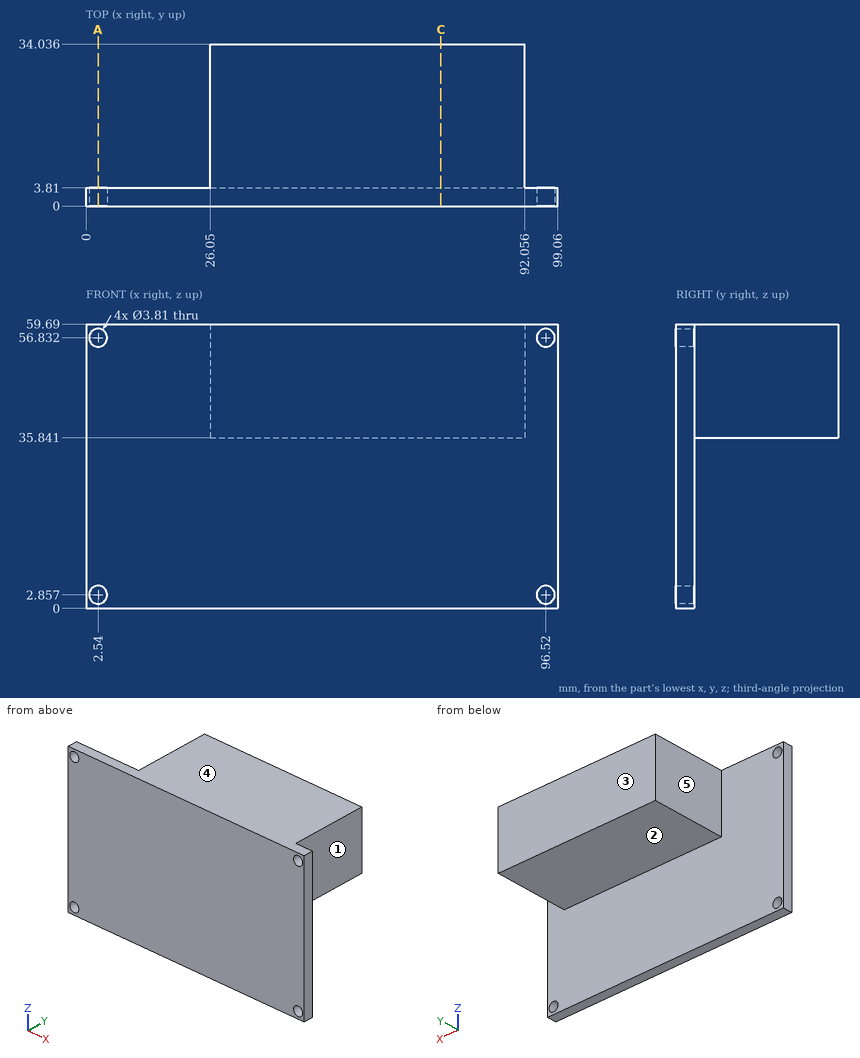
The figure shows three views and two pictorial views of one solid part (mm, origin at its lowest corner). Answer the questions. A direction names the side the tool comes from. Round coordinates to 2 decimals unless told otherwise and drop trailing zeros. Write each loop counter-clockwise with the first axis right and the second up, starting at its lowest first coordinate (ties: lowest second). Pieces come first, ordered by that corner, then holes. Notation, with made-up numbers: (11, 86.25) - (51, 86.25) arc R34 cw to (51, 117.25) - close; hole circle Ø1 at (75.5, 64). An arc over 180 degrees is marked (long way). Answer in a Markdown table with one row per item. Add a question column.
1. Find the intervals of material crossed by line 1 along Z through (x, y) = (2.54, 2.2); line 2 along Z through (x, y) = (2, 1) (1 decimal); line 3 along Y through (x, z) = (45, 17.5), in increasing order. Write a range as from..to.
2. Given pin 1 (3 mm diameter, centred on x = 96.52, z = 2.86, fed in from -Y); pin 2 (12 mm diameter, centred on y = 19.5, z = 46.5, fed in from +X); pin 3 (4.5 mm diameter, centred on x = 96.52, z = 56.83, fed in from +Y); pin 4 (4 mm diameter, centred on y = 10, z = 50.5, fed in from -X), each flat-ended and moving along its own axis, determine where each tip first touches the part or whether it passes through.
3. For the marked faces 1, 2, 3, 4 and 5, determine the directions among +Z, -Z, +X, -X, +Y, -Y from which every point of the face is accessible in a straight line to the end or side of a thin tool.
4. A cutting plane is placed at A-A, the plane x = 2.54. Determine the outline of the cut face in (y, z).
5. A cutting plane is placed at C-C, the plane x = 74.5. Determine the outline of the cut face in (y, z) (1 decimal).
Worked out:
| question | item | result |
|---|---|---|
| 1 | line 1 | 0..0.95, 4.76..54.93, 58.74..59.69 |
| 1 | line 2 | 0..1, 4.7..55, 58.7..59.7 |
| 1 | line 3 | 0..3.81 |
| 2 | pin 1 | through |
| 2 | pin 2 | x = 92.06 |
| 2 | pin 3 | y = 3.81 |
| 2 | pin 4 | x = 26.05 |
| 3 | face 1 | +Z, -Z, +X, +Y |
| 3 | face 2 | -Z, +X, -X, +Y |
| 3 | face 3 | +Z, -Z, +X, -X, +Y |
| 3 | face 4 | +Z, +X, -X, +Y, -Y |
| 3 | face 5 | +Z, -Z, -X, +Y |
| 4 | outline | (0, 0) - (3.81, 0) - (3.81, 0.95) - (0, 0.95) - close; (0, 4.76) - (3.81, 4.76) - (3.81, 54.93) - (0, 54.93) - close; (0, 58.74) - (3.81, 58.74) - (3.81, 59.69) - (0, 59.69) - close |
| 5 | outline | (0, 0) - (3.8, 0) - (3.8, 35.8) - (34, 35.8) - (34, 59.7) - (0, 59.7) - close |
